Read the model definition and answer for the solid it produces. Units are mm, in the model's axes. Face numbers are marked on the shaded views. A direction names the side the tool comes from. Coordinates: 2 decimals unless noted, no trailing zeros. Order: outer loops, then holes, each group sorted by start corner. A loop starts at its lowest first (then second) coordinate and runs counter-clockwise, first axis right, second up. Notation, with made-up numbers: (-34, -2) - (17, -2) arc R26 cw to (17, 36) - close; hole circle Ø3 at (-18.75, 62). An arc over 180 degrees is marked (long way). Answer as a JSON object with one key per item and string values. Group by question number.
from build123d import *

# Parameters (mm, degrees)
BOSS_EXTRUDE1_DEPTH = 5
CUT_EXTRUDE1_DEPTH  = 2.5
SKETCH5_R           = 1.6
CUT_EXTRUDE2_DEPTH  = 13.5


with BuildPart() as part:
    # Sketch2 → Boss-Extrude1 (new body)
    with BuildSketch(Plane(origin=(0, 0, 0), x_dir=(1, 0, 0), z_dir=(0, 1, 0))):
        Polygon((-5, 0), (-7.5, 0), (-7.5, 3.5), (-5, 3.5), (5, 3.5), (7.5, 3.5), (7.5, 0), (5, 0), (5, -3.5), (-5, -3.5), align=None)
    extrude(amount=BOSS_EXTRUDE1_DEPTH)

    # Sketch3 → Cut-Extrude1 (cut)
    with BuildSketch(Plane.XZ):
        Polygon((3.175426481, 0), (1.58771324, 2.75), (-1.58771324, 2.75), (-3.175426481, 0), (-1.58771324, -2.75), (1.58771324, -2.75), align=None)
    extrude(amount=-CUT_EXTRUDE1_DEPTH, mode=Mode.SUBTRACT)

    # Sketch4 → Revolve1 (revolve)
    with BuildSketch(Plane.XY):
        Polygon((1.6, 5), (1.6, 15), (2.25, 15), (2.25, 10), (3.25, 10), (3.25, 5), align=None)
    revolve(axis=Axis((0, 0, 0), (0, 1, 0)))

    # Sketch5 → Cut-Extrude2 (cut, through all)
    with BuildSketch(Plane.XZ.offset(-2.5)):
        Circle(SKETCH5_R)
    extrude(amount=-CUT_EXTRUDE2_DEPTH, mode=Mode.SUBTRACT)


solid = part.part
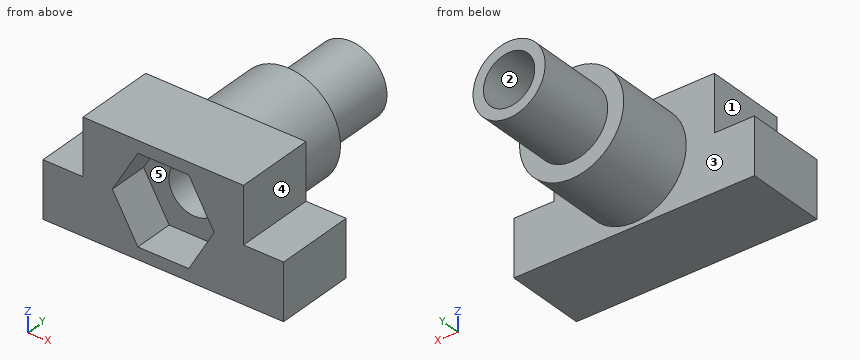
1. A cutting plane is placed at A-A on x = 0. Write down the section's boundary in (y, z), and give its area (4 significant figures).
2. A cutting plane is placed at C-C on z = 1. Write down the section's boundary in (x, y).
3. A cutting plane is placed at B-B on y = 2. Write down the section's boundary in (x, z).
4. Straight lines are drawn through the part: L1, parallel to Z at x = 0, y = 6.75; L2, parallel to X at y = 12.5, z = 0. For each, find the intervals that lie inside material, in ascending order.
5. For the marked faces 1, 2, 3, 4 and 5, determine the directions among +Z, -Z, +X, -X, +Y, -Y from which every point of the face is accessible in a straight line to the end or side of a thin tool.
6. Given pin 1 (1.6 mm diameter, centred on x = 1.5, z = 0, fed in from -Y); pin 2 (0.8 mm diameter, centred on x = 6, y = 1.5, fed in from +Z), each flat-ended and moving along its own axis, determine where each tip first touches the part or whether it passes through.
7. A cutting plane is placed at D-D on z = 3. Write down the section's boundary in (x, y), and give its area (3 significant figures).
Derived:
{
 "1": {"outline": "(0, -3.5) - (5, -3.5) - (5, -3.25) - (10, -3.25) - (10, -2.25) - (15, -2.25) - (15, -1.6) - (2.5, -1.6) - (2.5, -2.75) - (0, -2.75) - close; (0, 2.75) - (2.5, 2.75) - (2.5, 1.6) - (15, 1.6) - (15, 2.25) - (10, 2.25) - (10, 3.25) - (5, 3.25) - (5, 3.5) - (0, 3.5) - close", "area": "36.25 mm2"},
 "2": {"outline": "(-5, 0) - (-2.6, 0) - (-2.6, 2.5) - (-1.25, 2.5) - (-1.25, 15) - (-2.02, 15) - (-2.02, 10) - (-3.09, 10) - (-3.09, 5) - (-5, 5) - close; (1.25, 2.5) - (2.6, 2.5) - (2.6, 0) - (5, 0) - (5, 5) - (3.09, 5) - (3.09, 10) - (2.02, 10) - (2.02, 15) - (1.25, 15) - close"},
 "3": {"outline": "(-7.5, -3.5) - (7.5, -3.5) - (7.5, 0) - (5, 0) - (5, 3.5) - (-5, 3.5) - (-5, 0) - (-7.5, 0) - close; hole (-3.18, 0) - (-1.59, -2.75) - (1.59, -2.75) - (3.18, 0) - (1.59, 2.75) - (-1.59, 2.75) - close"},
 "4": {"L1": "z = -3.25 to -1.6, 1.6 to 3.25", "L2": "x = -2.25 to -1.6, 1.6 to 2.25"},
 "5": {"face 1": "+Z, -X, +Y, -Y", "face 2": "+Y, -Y", "face 3": "+Y", "face 4": "+Z, +X, +Y, -Y", "face 5": "-Y"},
 "6": {"pin 1": "stops at y = 2.5", "pin 2": "stops at z = 0"},
 "7": {"outline": "(-5, 0) - (5, 0) - (5, 5) - (1.25, 5) - (1.25, 10) - (-1.25, 10) - (-1.25, 5) - (-5, 5) - close", "area": "62.5 mm2"}
}
